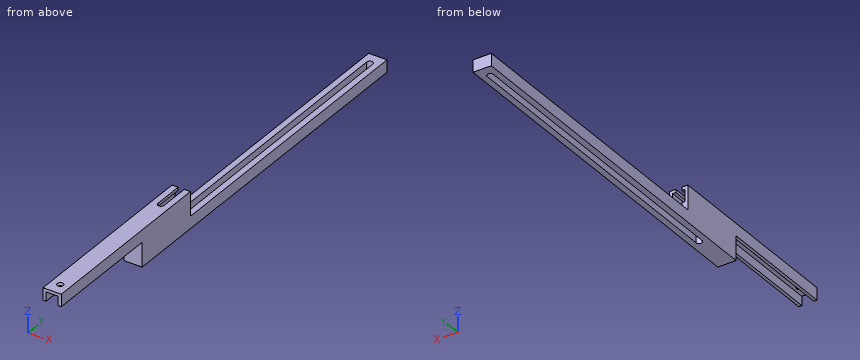
from build123d import *

# Parameters (mm, degrees)
F0_W     = 19.05
F0_H     = 38.1
F0_W_2   = 12.7
F0_H_2   = 12.7
F1_DEPTH = 508
F2_R     = 3.175
F3_DEPTH = 63.5
F4_W     = 306.7244030911
F4_H     = 25.4
F4_W_2   = 126.1607544422
F5_DEPTH = 25.4


with BuildPart() as f1:
    # F0 (on Front) → F1 (new body)
    with BuildSketch(Plane.XZ):
        with Locations((-6.35, -3.175)):
            Rectangle(F0_W, F0_H)
        with Locations((-6.35, 6.35)):
            Rectangle(F0_W_2, F0_H_2, mode=Mode.SUBTRACT)
    extrude(amount=F1_DEPTH)

    # F2 (on Top) → F3 (cut, symmetric)
    with BuildSketch(Plane.XY):
        with BuildLine():
            Line((-3.175, -254), (-3.175, -12.7))
            ThreePointArc((-3.175, -12.7), (-6.35, -9.525), (-9.525, -12.7))
            Line((-9.525, -12.7), (-9.525, -254))
            Line((-9.525, -254), (-9.525, -338.2622301579))
            ThreePointArc((-9.525, -338.2622301579), (-6.35, -341.4372301579), (-3.175, -338.2622301579))
            Line((-3.175, -338.2622301579), (-3.175, -254))
        make_face()
        with Locations((-6.35, -495.3)):
            Circle(F2_R)
    extrude(amount=F3_DEPTH, both=True, mode=Mode.SUBTRACT)

    # F4 (on face) → F5 (cut)
    with BuildSketch(Plane(origin=(-15.875, 0, 0), x_dir=(0, -1, 0), z_dir=(-1, 0, 0))):
        with Locations((153.3622015456, 3.175)):
            Rectangle(F4_W, F4_H)
        with Locations((444.9196227789, -9.525)):
            Rectangle(F4_W_2, F4_H)
    extrude(amount=-F5_DEPTH, mode=Mode.SUBTRACT)


solid = f1.part
For this review, take the finished solid that the model builds, in its own axes (mm). Give positions to 0.01 mm unless a question says otherwise; leave off trailing zeros. Loops run counter-clockwise (first coordinate to the right, second up) from the corner with the lowest first, then second, coordinate; pieces in that order, holes last. Notation, with made-up numbers: M 27,83 L 33,83 A27 ccw 33,109 Z; hole C 77.25,76.5 d11. An arc over 180 degrees is marked long. Answer as a JSON object with one key per item and string values. Group by question number.
Q1. Add section C-C on x = -6.35. Give the boundary of the cut face in (y, z) (3 decimals), and give its area (3 significant figures).
Q2. Add section A-A on y = -330. Give the boundary of the cut face in (x, z) (3 decimals), and give its area (3 significant figures).
Q3. Insertion check: P1, Ø5.5, axis at x = -10.5, z = -8, coming from the -Y side; P2, Ø10, axis at x = -4, y = -392.5, coming from the -Z side (3 decimals); P3, Ø3, axis at x = -1, z = 0, coming from the +Y side. Each pin has a flat end and moves straight along its axis. Give the tip position at first contact, or say it passes through.
Q4. Add section B-B on z = 8.5. Give the boundary of the cut face in (x, y) (3 decimals), and give its area (3 significant figures).
Q5. For probe 1 along X at (y, z) = (-209, -16.5) (3 decimals); probe 2 along X at (y, z) = (-351.5, 5) (3 decimals); probe 3 along Z at (x, y) = (-3, -209.5) (3 decimals), list the stretches that pass through material, from the lowest coordinate up. Write a range as [from, to].
Q6. Add section D-D on y = -205. Give the boundary of the cut face in (x, z) (3 decimals), and give its area (3 significant figures).
Checked values:
{
 "1": {"outline": "M -508,12.7 L -498.475,12.7 L -498.475,15.875 L -508,15.875 Z; M -492.125,12.7 L -341.437,12.7 L -341.437,15.875 L -492.125,15.875 Z; M -381.839,-22.225 L -341.437,-22.225 L -341.437,0 L -381.839,0 Z; M -9.525,-22.225 L 0,-22.225 L 0,-9.525 L -9.525,-9.525 Z", "area": "1,530 mm²"},
 "2": {"outline": "M -15.875,-22.225 L -9.525,-22.225 L -9.525,0 L -12.7,0 L -12.7,12.7 L -9.525,12.7 L -9.525,15.875 L -15.875,15.875 Z; M -3.175,-22.225 L 3.175,-22.225 L 3.175,15.875 L -3.175,15.875 L -3.175,12.7 L 0,12.7 L 0,0 L -3.175,0 Z", "area": "403 mm²"},
 "3": {"P1": "y = -381.84", "P2": "z = 3.175", "P3": "y = -306.72"},
 "4": {"outline": "M -15.875,-508 L -12.7,-508 L -12.7,-306.724 L -15.875,-306.724 Z; M 0,-508 L 3.175,-508 L 3.175,-306.724 L 0,-306.724 Z", "area": "1,280 mm²"},
 "5": {"probe 1": "[-15.875, -9.525], [-3.175, 3.175]", "probe 2": "[-15.875, -12.7], [0, 3.175]", "probe 3": "[-22.225, -9.525]"},
 "6": {"outline": "M -15.875,-22.225 L -9.525,-22.225 L -9.525,-9.525 L -15.875,-9.525 Z; M -3.175,-22.225 L 3.175,-22.225 L 3.175,-9.525 L -3.175,-9.525 Z", "area": "161 mm²"}
}
